Autodesk Inventor part; units mm, degrees
ref_plane "YZ Plane" through (0, 0, 0) normal (1, 0, 0) x (0, 1, 0)
ref_plane "XZ Plane" through (0, 0, 0) normal (0, 1, 0) x (-1, 0, 0)
ref_plane "XY Plane" through (0, 0, 0) normal (0, 0, 1) x (1, 0, 0)
sketch "Sketch2" plane through (0, 0, 0) normal (0, 1, 0) x (-1, 0, 0)
  line L0 (0, 0) -> (-36, 0)
  line L1 (-36, 0) -> (-36, -100)
  line L2 (-36, -100) -> (0, -100)
  line L3 (0, -100) -> (0, 0)
  line L4 (-36, 0) -> (-36, -20)
  line L5 (-36, -20) -> (0, -20)
  line L6 (-36, -100) -> (-36, -80)
  line L7 (-36, -80) -> (-36, -61.7109)
  line L8 (0, -61.7109) -> (0, -80)
  line L9 (-36, -80) -> (-36, -70)
  line L10 (-36, -70) -> (0, -70)
  line L11 (0, -80) -> (-36, -80)
  line L12 (0, -70) -> (0, -80)
  line L13 (0, -70) -> (-5, -70)
  line L14 (-5, -70) -> (-5, -80)
  line L15 (-36, -20) -> (-36, -30)
  line L16 (-36, -30) -> (0, -30)
  line L17 (0, -20) -> (-5, -20)
  line L18 (-5, -20) -> (-5, -30)
  line L19 (-36, -80) -> (-31, -80)
  line L20 (-31, -80) -> (-31, -70)
  line L21 (-31, -30) -> (-31, -20)
  line L22 (-18, 0) -> (-18, -15)
  circle A0 centre (-18, -15) radius 12
  line L23 (-18, -15) -> (-18, -45.5)
  line L24 (-18, -45.5) -> (-18, -86)
  line L25 (-18, -15) -> (-18, -43.5)
  circle A1 centre (-18, -43.5) radius 5.05
  line L26 (-18, -43.5) -> (-18, -82)
  circle A2 centre (-18, -82) radius 5.05
  dimension "d0" = 36
  dimension "d1" = 100
  dimension "d2" = 20
  dimension "d3" = 20
  dimension "d4" = 10
  dimension "d5" = 5
  dimension "d6" = 10
  dimension "d7" = 5
  dimension "d8" = 5
  dimension "d9" = 15
  dimension "d10" = 24
  dimension "d17" = 28.5
  dimension "d18" = 10.1
  dimension "d19" = 38.5
  dimension "d20" = 10.1
extrude "Extrusion1" add sketch "Sketch2" along normal blind 5 contours L3 L5 A0 L22 L0 | L22 A0 L5 L1 L0 | L3 L10 L24 A1 L23 L16 | L18 L16 L23 A0 L5 | A0 L23 L16 L21 L5 | L16 L23 A1 L24 L10 L1 | L3 L2 L1 L11 A2 | L14 L11 A2 L24 L10 | L24 A2 L11 L20 L10
equation "\"BendRadius\" = Thickness"
equation "\"BendReliefWidth\" = Thickness"
equation "\"BendReliefDepth\" = 0.5 * Thickness"
equation "\"CornerReliefSize\" = 4 * Thickness"
equation "\"MinimumRemnant\" = 2 * Thickness"
equation "\"TransitionRadius\" = BendRadius"
equation "\"JacobiRadiusSize\" = BendRadius"
equation "\"GapSize\" = Thickness"
Input: part model. Units: mm. Frame: model coordinates. A direction names the side the tool comes from. Round coordinates to 2 decimals unless told otherwise and drop trailing zeros. Order: outer loops, then holes, each group sorted by start corner. A loop starts at its lowest first (then second) coordinate and runs counter-clockwise, first axis right, second up. Notation, with made-up numbers: (-15.75, -22) - (24.25, -22) arc R21 ccw to (24.25, 15) - close; hole circle Ø2 at (-27, 47.5). An arc over 180 degrees is marked (long way). One line per question, with ' | ' between items. Start each with the question number.
1) Cut plane D-D, the plane x = 24. Return the cut outline in (y, z).
2) Cut plane A-A, the plane x = 18. Return the cut outline in (y, z), then the cut area to 3 significant figures.
3) Cut plane B-B, the plane z = -43.5. Return the cut outline in (x, y), then the cut area to 4 significant figures.
4) Contact query for flat-ended pins moving along their axis: P1, Ø2.5, axis at y = 3.5, z = -73.5, coming from the +X side; P2, Ø6, axis at x = 18, z = -82, coming from the -Y side. Output: stop coordinate, or through.
5) Ray query, probe 1 along Z at (x, y) = (18, 3.8); probe 2 along X at (y, z) = (2.4, -15); probe 3 along X at (y, z) = (3.75, -82). Return the intervals inside material, ascending.
6) Cut plane C-C, the plane y = 1.9. Return the cut outline in (x, z), then the cut area to 3 significant figures.
7) Set-up query: faces 1 (the flat face through (31, 2, -25)), 2 (the flat face through (5, 2, -75)), 3 (the flat face through (0, 2, -10)). Return all of +Z, -Z, +X, -X, +Y, -Y with unobstructed straight access to the full face (end or side cutting, diameter ignored); none if empty.
8) Pull-direction query (Z, two-part tool) for faces 4 (the flat face through (18, 0, -49)), 5 (the flat face through (18, 2, -100)), 6 (the cylindrical face through (6.554, 2.465, -18.604)); classes: +Z half, -Z half, draft (parallel to the pull), parting line (faces both ways), or undercut.
Worked out:
1) outline: (0, -100) - (5, -100) - (5, -25.39) - (0, -25.39) - close; (0, -4.61) - (5, -4.61) - (5, 0) - (0, 0) - close
2) outline: (0, -100) - (5, -100) - (5, -87.05) - (0, -87.05) - close; (0, -76.95) - (5, -76.95) - (5, -48.55) - (0, -48.55) - close; (0, -38.45) - (5, -38.45) - (5, -27) - (0, -27) - close; (0, -3) - (5, -3) - (5, 0) - (0, 0) - close | area: 279 mm^2
3) outline: (0, 0) - (12.95, 0) - (12.95, 5) - (0, 5) - close; (23.05, 0) - (36, 0) - (36, 5) - (23.05, 5) - close | area: 129.5 mm^2
4) P1: stops at x = 31 | P2: passes through
5) probe 1: z = -100 to -87.05, -76.95 to -48.55, -38.45 to -27, -3 to 0 | probe 2: x = 0 to 6, 30 to 36 | probe 3: x = 0 to 12.95, 23.05 to 36
6) outline: (0, -100) - (36, -100) - (36, -80) - (31, -80) - (31, -70) - (36, -70) - (36, -30) - (31, -30) - (31, -20) - (36, -20) - (36, 0) - (0, 0) - (0, -20) - (5, -20) - (5, -30) - (0, -30) - (0, -70) - (5, -70) - (5, -80) - (0, -80) - close; hole circle Ø24 at (18, -15); hole circle Ø10.1 at (18, -82); hole circle Ø10.1 at (18, -43.5) | area: 2,790 mm^2
7) face 1: +X, +Y, -Y | face 2: -X, +Y, -Y | face 3: +Z, -Z, -X, +Y, -Y
8) face 4: draft | face 5: -Z half | face 6: undercut
